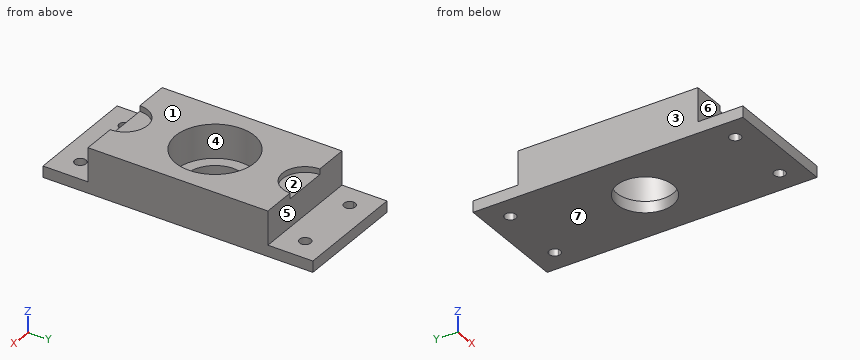
```python
from build123d import *

# Parameters (mm, degrees)
BOSS_EXTRUDE1_DEPTH = 25.4
SKETCH2_W           = 63.5
SKETCH2_H           = 25.4
CUT_EXTRUDE1_DEPTH  = 19.05
SKETCH3_R           = 15.875
CUT_EXTRUDE4_DEPTH  = 26.4
SKETCH5_R           = 22.225
SKETCH5_R_2         = 15.875
CUT_EXTRUDE6_DEPTH  = 19.05
SKETCH6_R           = 12.7
CUT_EXTRUDE7_DEPTH  = 3.175
BOSS_EXTRUDE2_DEPTH = 25.4
SKETCH9_W           = 19.05
SKETCH9_H           = 3.556
BOSS_EXTRUDE4_DEPTH = 35.56


with BuildPart() as part:
    # Sketch1 → Boss-Extrude1 (new body)
    with BuildSketch(Plane.XY):
        with BuildLine():
            Line((-19.05, -66.675), (-19.05, -76.2))
            Line((-19.05, -76.2), (19.05, -76.2))
            Line((19.05, -76.2), (19.05, -66.675))
            ThreePointArc((19.05, -66.675), (16.80493597, -61.25493597), (22.225, -63.5))
            Line((22.225, -63.5), (31.75, -63.5))
            Line((31.75, -63.5), (31.75, 63.5))
            Line((31.75, 63.5), (22.225, 63.5))
            ThreePointArc((22.225, 63.5), (16.80493597, 61.25493597), (19.05, 66.675))
            Line((19.05, 66.675), (19.05, 76.2))
            Line((19.05, 76.2), (-19.05, 76.2))
            Line((-19.05, 76.2), (-19.05, 66.675))
            ThreePointArc((-19.05, 66.675), (-16.80493597, 65.74506403), (-15.875, 63.5))
            ThreePointArc((-15.875, 63.5), (-19.05, 60.325), (-22.225, 63.5))
            Line((-22.225, 63.5), (-31.75, 63.5))
            Line((-31.75, 63.5), (-31.75, -63.5))
            Line((-31.75, -63.5), (-22.225, -63.5))
            ThreePointArc((-22.225, -63.5), (-19.05, -60.325), (-15.875, -63.5))
            ThreePointArc((-15.875, -63.5), (-16.80493597, -65.74506403), (-19.05, -66.675))
        make_face()
        with BuildLine():
            Line((-31.75, 76.2), (-31.75, 63.5))
            Line((-31.75, 63.5), (-22.225, 63.5))
            ThreePointArc((-22.225, 63.5), (-21.29506403, 65.74506403), (-19.05, 66.675))
            Line((-19.05, 66.675), (-19.05, 76.2))
            Line((-19.05, 76.2), (-31.75, 76.2))
        make_face()
        with BuildLine():
            Line((22.225, 63.5), (31.75, 63.5))
            Line((31.75, 63.5), (31.75, 76.2))
            Line((31.75, 76.2), (19.05, 76.2))
            Line((19.05, 76.2), (19.05, 66.675))
            ThreePointArc((19.05, 66.675), (21.29506403, 65.74506403), (22.225, 63.5))
        make_face()
        with BuildLine():
            Line((-31.75, -63.5), (-31.75, -76.2))
            Line((-31.75, -76.2), (-19.05, -76.2))
            Line((-19.05, -76.2), (-19.05, -66.675))
            ThreePointArc((-19.05, -66.675), (-21.29506403, -65.74506403), (-22.225, -63.5))
            Line((-22.225, -63.5), (-31.75, -63.5))
        make_face()
        with BuildLine():
            Line((19.05, -66.675), (19.05, -76.2))
            Line((19.05, -76.2), (31.75, -76.2))
            Line((31.75, -76.2), (31.75, -63.5))
            Line((31.75, -63.5), (22.225, -63.5))
            ThreePointArc((22.225, -63.5), (21.29506403, -65.74506403), (19.05, -66.675))
        make_face()
    extrude(amount=BOSS_EXTRUDE1_DEPTH)

    # Sketch2 → Cut-Extrude1 (cut)
    with BuildSketch(Plane.XY.offset(25.4)):
        with Locations((0, 63.5)):
            Rectangle(SKETCH2_W, SKETCH2_H)
        with Locations((0, -63.5)):
            Rectangle(SKETCH2_W, SKETCH2_H)
    extrude(amount=-CUT_EXTRUDE1_DEPTH, mode=Mode.SUBTRACT)

    # Sketch3 → Cut-Extrude4 (cut, through all)
    with BuildSketch(Plane.XY.offset(25.4)):
        Circle(SKETCH3_R)
    extrude(amount=-CUT_EXTRUDE4_DEPTH, mode=Mode.SUBTRACT)

    # Sketch5 → Cut-Extrude6 (cut)
    with BuildSketch(Plane.XY.offset(25.4)):
        Circle(SKETCH5_R)
        Circle(SKETCH5_R_2, mode=Mode.SUBTRACT)
    extrude(amount=-CUT_EXTRUDE6_DEPTH, mode=Mode.SUBTRACT)

    # Sketch6 → Cut-Extrude7 (cut)
    with BuildSketch(Plane.XY.offset(25.4)):
        with Locations((0, -50.8)):
            Circle(SKETCH6_R)
        with Locations((0, 50.8)):
            Circle(SKETCH6_R)
    extrude(amount=-CUT_EXTRUDE7_DEPTH, mode=Mode.SUBTRACT)


with BuildPart() as body_2:
    # Sketch7 → Boss-Extrude2 (new body)
    with BuildSketch(Plane.ZY.offset(31.75)):
        Polygon((0, 123.19), (19.05, 123.19), (19.05, -50.8), (6.35, -50.8), (6.35, -76.2), (0, -76.2), align=None)
    extrude(amount=BOSS_EXTRUDE2_DEPTH)

    # Sketch9 → Boss-Extrude4 (add)
    with BuildSketch(Plane.ZY.offset(57.15)):
        with Locations((9.525, 121.412)):
            Rectangle(SKETCH9_W, SKETCH9_H)
        with Locations((9.525, 110.236)):
            Rectangle(SKETCH9_W, SKETCH9_H)
    extrude(amount=BOSS_EXTRUDE4_DEPTH)


solid = part.part
```
The model under review builds one solid part; all positions refer to its coordinate system, in mm. Face numbers are marked on the shaded views. A direction names the side the tool comes from. Round coordinates to 2 decimals unless told otherwise and drop trailing zeros. Loops run counter-clockwise (first coordinate to the right, second up) from the corner with the lowest first, then second, coordinate; pieces in that order, holes last. Notation, with made-up numbers: (-18.5, 56.5) -> (21.5, 56.5) arc R29 ccw to (21.5, 93.5) -> close; hole circle Ø8 at (50, -18). An arc over 180 degrees is marked (long way). Answer as a JSON object with one key per item and string values. Group by question number.
1) We need section A-A on x = -4.5. Write out the cut boundary in (y, z) (3 decimals).
2) We need section D-D on x = 26. Write out the cut boundary in (y, z), then the cut area to 3 significant figures.
3) Mouldability with a two-part tool opening along X and no side actions: class the marked faces 1, 2, 3 and 4 as released by +X, released by -X, zero draft, split by the parting line, or undercut.
4) For the marked faces 5, 6 and 7, list the 3-axis set-ups (+Z, -Z, +X, -X, +Y, -Y) from which the entire face can be reached by the end or side of a thin tool; tool diameter is ignored.
5) For pin 1 Ø1.5 at (x, z) = (11, 14.5) entering from +Y; pin 2 Ø4 at (x, y) = (19.05, 63.5) entering from -Z; pin 3 Ø12 at (x, y) = (-2, -11.5) entering from +Z; pin 4 Ø4 at (x, y) = (4.5, -44) entering from +Z (3 decimals), all flat-tipped, find the tip position at first contact; note any pin that passes through.
6) We need section C-C on y = -11.5. Write out the cut boundary in (x, z), then the cut area to 3 significant figures.
7) We need section B-B on z = 10.5. Write out the cut boundary in (x, y) (3 decimals), then the cut area to 3 significant figures.
8) For line 1 (Y direction, x = 19.05, z = 3) (3 decimals); line 2 (Y direction, x = 19.5, z = 5.5); line 3 (X direction, y = 63.5, z = 2.75) (3 decimals), list the stretches that pass through material, from the lowest coordinate up. Write a range as [from, to].
Result set:
{
 "1": {"outline": "(-76.2, 0) -> (-15.224, 0) -> (-15.224, 6.35) -> (-21.765, 6.35) -> (-21.765, 25.4) -> (-38.924, 25.4) -> (-38.924, 22.225) -> (-50.8, 22.225) -> (-50.8, 6.35) -> (-76.2, 6.35) -> close; (15.224, 0) -> (76.2, 0) -> (76.2, 6.35) -> (50.8, 6.35) -> (50.8, 22.225) -> (38.924, 22.225) -> (38.924, 25.4) -> (21.765, 25.4) -> (21.765, 6.35) -> (15.224, 6.35) -> close"},
 "2": {"outline": "(-76.2, 0) -> (76.2, 0) -> (76.2, 6.35) -> (50.8, 6.35) -> (50.8, 25.4) -> (-50.8, 25.4) -> (-50.8, 6.35) -> (-76.2, 6.35) -> close", "area": "2,900 mm²"},
 "3": {"face 1": "zero draft", "face 2": "undercut", "face 3": "released by -X", "face 4": "undercut"},
 "4": {"face 5": "+Z, +X, -X, +Y", "face 6": "+Z, +X, -X, -Y", "face 7": "-Z, +X, -X, +Y, -Y"},
 "5": {"pin 1": "y = 50.8", "pin 2": "through", "pin 3": "z = 6.35", "pin 4": "z = 22.225"},
 "6": {"outline": "(-31.75, 0) -> (-10.94, 0) -> (-10.94, 6.35) -> (-19.02, 6.35) -> (-19.02, 25.4) -> (-31.75, 25.4) -> close; (10.94, 0) -> (31.75, 0) -> (31.75, 25.4) -> (19.02, 25.4) -> (19.02, 6.35) -> (10.94, 6.35) -> close", "area": "749 mm²"},
 "7": {"outline": "(-31.75, -50.8) -> (31.75, -50.8) -> (31.75, 50.8) -> (-31.75, 50.8) -> close; hole circle Ø44.45 at (0, 0)", "area": "4,900 mm²"},
 "8": {"line 1": "[-76.2, -66.675], [-60.325, 60.325], [66.675, 76.2]", "line 2": "[-76.2, -66.64], [-60.36, 60.36], [66.64, 76.2]", "line 3": "[-31.75, -22.225], [-15.875, 15.875], [22.225, 31.75]"}
}
